The listing builds one solid part. Answer for the finished solid, in the listing's coordinates (mm). Round coordinates to 2 decimals unless told otherwise and drop trailing zeros. Write each loop counter-clockwise with the first axis right and the second up, starting at its lowest first coordinate (ties: lowest second). Pieces come first, ordered by that corner, then holes.
Item 1: Find the intervals of material crossed by probe 1 along X at (y, z) = (2.45, -70); probe 2 along X at (y, z) = (2.45, -10); probe 3 along Z at (x, y) = (-20.5, 1.4), in increasing order.
Item 2: Find section B-B on x = -4. Give the vertices of the cut face in (y, z).
Item 3: Find section D-D on z = -70. Give the vertices of the cut face in (x, y), then the cut area to 3 significant figures.
Item 4: Find section A-A on z = -10. Give the vertices of the cut face in (x, y).
Item 5: This flat-tipped pin is pushed along its axis until it touches: pin 1 (1 mm diameter, centred on x = 19, z = -32.5, fed in from +Y). Where does it stop, or does it pass through?
Item 6: Find section C-C on y = 2.8. Give the vertices of the cut face in (x, z), then the cut area to 3 significant figures.
```python
from build123d import *

# Parameters (mm, degrees)
BOSS_EXTRUDE1_DEPTH = 6
SKETCH2_R           = 2.5
SKETCH2_W           = 42
SKETCH2_H           = 42
CUT_EXTRUDE1_DEPTH  = 96.876222287


with BuildPart() as part:
    # Sketch1 → Boss-Extrude1 (new body)
    with BuildSketch(Plane(origin=(0, 0, 0), x_dir=(1, 0, 0), z_dir=(0, 1, 0))):
        Polygon((0, 0), (-52.5, 0), (-52.5, 80), (52.5, 80), (52.5, 0), align=None)
    extrude(amount=BOSS_EXTRUDE1_DEPTH)

    # Sketch2 → Cut-Extrude1 (cut, through all)
    with BuildSketch(Plane(origin=(0, 6, 0), x_dir=(1, 0, 0), z_dir=(0, 1, 0))):
        with Locations(Location((-42.5, 70, 0), (0, 0, 270))):
            Circle(SKETCH2_R)
        with Locations(Location((42.5, 70, 0), (0, 0, 270))):
            Circle(SKETCH2_R)
        with Locations(Location((42.5, 10, 0), (0, 0, 270))):
            Circle(SKETCH2_R)
        with Locations(Location((0, 10, 0), (0, 0, 270))):
            Circle(SKETCH2_R)
        with Locations(Location((-42.5, 10, 0), (0, 0, 270))):
            Circle(SKETCH2_R)
        with Locations((0, 41)):
            Rectangle(SKETCH2_W, SKETCH2_H)
    extrude(amount=-CUT_EXTRUDE1_DEPTH, mode=Mode.SUBTRACT)


solid = part.part
```
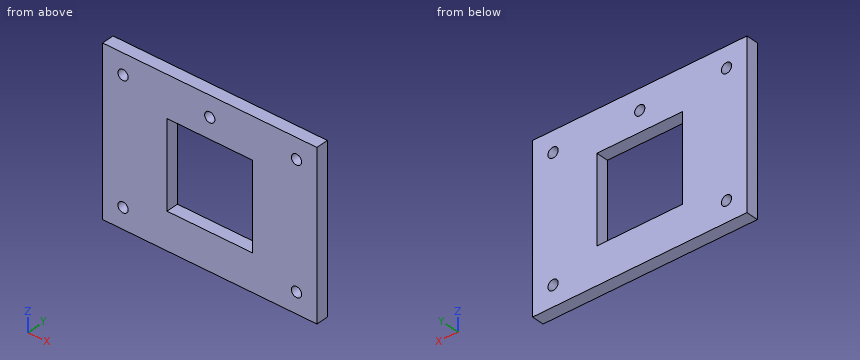
Check values:
1. probe 1: x = -52.5 to -45, -40 to 40, 45 to 52.5
1. probe 2: x = -52.5 to -45, -40 to -2.5, 2.5 to 40, 45 to 52.5
1. probe 3: z = -80 to -62, -20 to 0
2. outline: (0, -80) - (6, -80) - (6, -62) - (0, -62) - close; (0, -20) - (6, -20) - (6, 0) - (0, 0) - close
3. outline: (-52.5, 0) - (-45, 0) - (-45, 6) - (-52.5, 6) - close; (-40, 0) - (40, 0) - (40, 6) - (-40, 6) - close; (45, 0) - (52.5, 0) - (52.5, 6) - (45, 6) - close
3. area: 570 mm2
4. outline: (-52.5, 0) - (-45, 0) - (-45, 6) - (-52.5, 6) - close; (-40, 0) - (-2.5, 0) - (-2.5, 6) - (-40, 6) - close; (2.5, 0) - (40, 0) - (40, 6) - (2.5, 6) - close; (45, 0) - (52.5, 0) - (52.5, 6) - (45, 6) - close
5. pin 1: passes through
6. outline: (-52.5, -80) - (52.5, -80) - (52.5, 0) - (-52.5, 0) - close; hole circle Ø5 at (-42.5, -70); hole circle Ø5 at (-42.5, -10); hole (-21, -62) - (21, -62) - (21, -20) - (-21, -20) - close; hole circle Ø5 at (0, -10); hole circle Ø5 at (42.5, -70); hole circle Ø5 at (42.5, -10)
6. area: 6,540 mm2
